Could you check a few things on this model? Use its own coordinates, in mm. Face numbers are marked on the shaded views. A direction names the side the tool comes from. Coordinates: 2 decimals unless noted, no trailing zeros. Loops run counter-clockwise (first coordinate to the right, second up) from the corner with the lowest first, then second, coordinate; pieces in that order, holes last. Notation, with made-up numbers: M 1,62 L 29,62 A38 cw 29,100 Z; hole C 54,-1.75 d7. An arc over 180 degrees is marked long. Use one line per item in the form item = value. Start each with the question number.
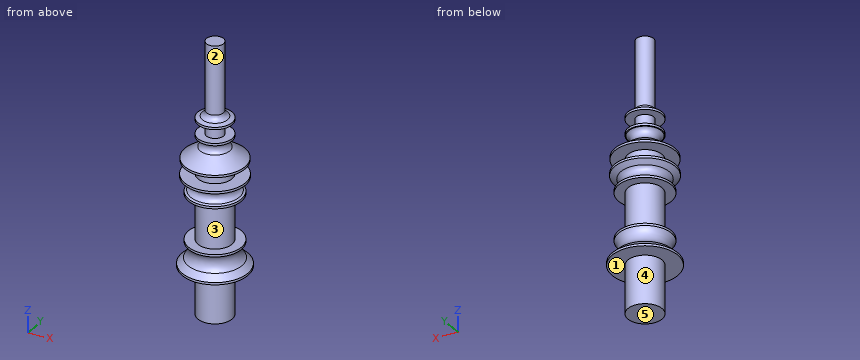
```python
from build123d import *

# Parameters (mm, degrees)
SKETCH1_R           = 14.999999999999998
BOSS_EXTRUDE1_DEPTH = 235.00000000000006
FILLET2_R           = 10
SKETCH4_W           = 104.26000000000013
SKETCH4_H           = 22.69462593232808
SKETCH10_R          = 15
BOSS_EXTRUDE2_DEPTH = 10
SCALE1_SCALE        = 1.9329
BOSS_EXTRUDE3_START = 40
SKETCH11_R          = 28.993500000000004
BOSS_EXTRUDE3_DEPTH = 40
FILLET3_R           = 10
FILLET5_R           = 10
FILLET6_R           = 10
FILLET7_R           = 10
SCALE2_SCALE        = 1.5
SKETCH12_R          = 43.49025000000001
CUT_EXTRUDE1_DEPTH  = 33.369805
SKETCH13_R          = 43.49025000000001
CUT_EXTRUDE2_DEPTH  = 20


with BuildPart() as part:
    # Sketch1 → Boss-Extrude1 (new body)
    with BuildSketch(Plane.XY):
        Circle(SKETCH1_R)
    extrude(amount=BOSS_EXTRUDE1_DEPTH)

    # Sketch2 → Revolve1 (revolve)
    with BuildSketch(Plane(origin=(0, 0, 0), x_dir=(1, 0, 0), z_dir=(0, 1, 0))):
        Polygon((0, -112.54820823836592), (0, -13.4987966999347), (11.119928350948882, -13.4987966999347), (11.119928350948882, -39.9), (15.000000000000005, -39.9), (28.84535837615048, -39.89999999999999), (28.845358376150482, -41.9), (16.269055666837332, -53.905209320131334), (23.203846346706012, -60.84), (23.203846346706015, -62.84), (7.5, -62.84), (7.4999999999999964, -102.74), (23.203846346706012, -102.74), (23.203846346706012, -104.74), (7.499999999999994, -112.54820823836592), align=None)
    revolve(axis=Axis((0, 0, 112.54820823836592), (0, 0, -1)))

    # Fillet2
    # the kernel refuses this fillet: 10 mm, written as the material it adds along each edge
    with BuildSketch(Plane(origin=(0, 0, 53.905209320131334), x_dir=(1, 0, 0), z_dir=(0, 1, 0))) as fillet2_piece_1:
        with BuildLine():
            CenterArc((30.57076321680232, -0.17250291395021122), FILLET2_R, 133.66910726980632, 88.8805373351795)
            Line((23.665838203316056, 7.060892592873103), (23.527739703046333, 7.205560503009572))
            Line((23.527739703046333, 7.205560503009572), (16.130957166567608, 0.1446679101364694))
            Line((16.130957166567608, 0.1446679101364694), (16.127634310600023, -0.14142135623730923))
            ThreePointArc((16.127634310600023, -0.14142135623730923), (19.595029650534364, -3.608816696171644), (23.05650800930409, -7.070036435187042))
            Line((23.05650800930409, -7.070036435187042), (23.203846346706015, -6.934790679868669))
        make_face()
    revolve(axis=Axis((0, 0, 53.905209320131334), (0, 0, -1)))
    with BuildSketch(Plane(origin=(0, 0, 108.81908605423119), x_dir=(1, 2.8e-16, 0), z_dir=(-2.8e-16, 1, 0))) as fillet2_piece_2:
        with BuildLine():
            CenterArc((14.999999999999998 + FILLET2_R, -FILLET2_R * 0.619575560585), FILLET2_R, 116.43731334282423, 63.56268665717579)
            Line((14.999999999999998 + FILLET2_R * 0.554781591202, FILLET2_R * 0.275846445214), (14.999999999999998 + FILLET2_R * 0.545877223026, FILLET2_R * 0.293754885329))
            Line((14.999999999999998 + FILLET2_R * 0.545877223026, FILLET2_R * 0.293754885329), (14.999999999999998 - FILLET2_R * 0.02, FILLET2_R * 0.0123915112117))
            Line((14.999999999999998 - FILLET2_R * 0.02, FILLET2_R * 0.0123915112117), (14.999999999999998 - FILLET2_R * 0.02, -FILLET2_R * 0.619575560585))
            Line((14.999999999999998 - FILLET2_R * 0.02, -FILLET2_R * 0.619575560585), (15, -FILLET2_R * 0.619575560585))
        make_face()
    revolve(axis=Axis((0, 0, 108.81908605423119), (0, 0, -1)))

    # Sketch3 → Revolve2 (revolve)
    with BuildSketch(Plane(origin=(0, 0, 0), x_dir=(0, 0, -1), z_dir=(1, 0, 0)), mode=Mode.PRIVATE) as revolve2_sk:
        Polygon((-130.74, 0), (-130.73999999999998, 14), (-128.73999999999995, 14), (-119.92783449185274, 1.1e-14), align=None)
    revolve(revolve2_sk.sketch.rotate(Axis((0, 1.1e-14, 119.92783449185274), (0, -1.02e-15, 1)), 90), axis=Axis((0, 1.1e-14, 119.92783449185274), (0, -1.02e-15, 1)))

    # Sketch4 → Cut-Revolve1 (revolve, cut)
    with BuildSketch(Plane(origin=(0, 0, 0), x_dir=(0, 0, -1), z_dir=(1, 0, 0)), mode=Mode.PRIVATE) as cut_revolve1_sk:
        with Locations((-182.87, -18.84731296616404)):
            Rectangle(SKETCH4_W, SKETCH4_H)
    revolve(cut_revolve1_sk.sketch.rotate(Axis((0, 0, 235.00000000000006), (0, 0, -1)), 90), axis=Axis((0, 0, 235.00000000000006), (0, 0, -1)), mode=Mode.SUBTRACT)

    # Sketch6 → Revolve4 (revolve)
    with BuildSketch(Plane(origin=(0, 0, 0), x_dir=(1, 0, 0), z_dir=(0, 1, 0))):
        Polygon((1.514e-14, -147.73999999999998), (1.829e-14, -173.48215721635322), (-14.999999999999986, -168.74), (-14.999999999999986, -166.74), (-7.589567298836239, -166.74), (-7.589567298836239, -154.73999999999998), (-14.999999999999986, -154.73999999999998), (-14.999999999999982, -152.73999999999998), align=None)
    revolve(axis=Axis((1.514e-14, 0, 147.73999999999998), (1.2e-16, 0, 1)))

    # Sketch8 → Revolve5 (revolve)
    with BuildSketch(Plane(origin=(0, 0, 0), x_dir=(0, 0, -1), z_dir=(1, 0, 0)), mode=Mode.PRIVATE) as revolve5_sk:
        Polygon((-152.73999999999998, 0), (-103.74000000000001, 0), (-117.74, 26.59546670677199), (-119.74, 26.59546670677199), (-119.74, 7.34766847272492), (-131.74, 7.34766847272492), (-131.74, 26.32680255189654), (-133.74, 26.32680255189654), align=None)
    revolve(revolve5_sk.sketch.rotate(Axis((0, 0, 152.73999999999998), (0, 0, -1)), 90), axis=Axis((0, 0, 152.73999999999998), (0, 0, -1)))

    # Sketch10 → Boss-Extrude2 (add)
    with BuildSketch(Plane.XY.offset(130.73999999999992)):
        with Locations(Location((0, 0, 0), (0, 0, 180))):
            Circle(SKETCH10_R)
    extrude(amount=BOSS_EXTRUDE2_DEPTH)


with BuildPart() as part_1:
    # Scale1: scaled about (0, 0, 88.197821602)
    add(part.part.scale(SCALE1_SCALE).moved(Location((0, 0, -82.27974777250581))))

    # Sketch11 → Boss-Extrude3 (add)
    with BuildSketch(Plane(origin=(0, 0, -82.27974777267455), x_dir=(-1, 0, 0), z_dir=(0, 0, -1)).offset(BOSS_EXTRUDE3_START)):
        Circle(SKETCH11_R)
    extrude(amount=-BOSS_EXTRUDE3_DEPTH)

    # Fillet3
    fillet3_edges = [part_1.edges().sort_by_distance(p)[0] for p in [
        (-29.95619321315706, -5.5e-15, 134.00840315083104),
    ]]
    fillet(fillet3_edges, radius=FILLET3_R)

    # Fillet5
    fillet5_edges = [part_1.edges().sort_by_distance(p)[0] for p in [
        (14.496749999993185, 4.19492707e-09, 248.4608560692405),
    ]]
    fillet(fillet5_edges, radius=FILLET5_R)

    # Fillet6
    # the kernel refuses this fillet: 10 mm, written as the material it adds along each edge
    with BuildSketch(Plane(origin=(-2.381562e-11, -3.695293e-11, 208.1191482274964), x_dir=(-1.0, 2.5486940639204283e-12, 0), z_dir=(-2.5486940639204283e-12, -1.0, 0))) as fillet6_piece_1:
        with BuildLine():
            CenterArc((24.364379904655884, 7.2517155656861405), FILLET6_R, 189.3328180990746, 62.23223307800339)
            Line((14.496750000023814, 5.630025069564624), (14.299397401931174, 5.597591259642201))
            ThreePointArc((14.299397401931174, 5.597591259642201), (14.296750000023817, 2.815012534782312), (14.296749999976186, 0))
            Line((14.296749999976186, 0), (14.433504446772817, -0.1897366596101051))
            Line((14.433504446772817, -0.1897366596101051), (21.13885669128414, -2.4248540744291063))
            Line((21.13885669128414, -2.4248540744291063), (21.202102244487506, -2.235117414819001))
        make_face()
    revolve(axis=Axis((-2.381562e-11, -3.695293e-11, 208.1191482274964), (0, 0, -1)))

    # Fillet7
    # the kernel refuses this fillet: 10 mm, written as the material it adds along each edge
    with BuildSketch(Plane(origin=(0, 0, 202.48912315793177), x_dir=(1, 2.8e-16, 0), z_dir=(-2.8e-16, 1, 0))) as fillet7_piece_1:
        with BuildLine():
            CenterArc((30.840499091800684, -0.5370158996013572), FILLET7_R, 125.81790747161939, 125.7471437054586)
            Line((24.988387693610907, 7.571793642074738), (24.40317655379193, 8.382674596242339))
            Line((24.40317655379193, 8.382674596242339), (13.911538860181022, 0.810880954167601))
            Line((13.911538860181022, 0.810880954167601), (13.509987009536637, -0.16216904961120804))
            ThreePointArc((13.509987009536637, -0.16216904961120804), (20.885874478501762, -8.813825782452454), (27.36199366561547, -10.972532178157024))
            Line((27.36199366561547, -10.972532178157024), (27.678221431632306, -10.023848880106499))
        make_face()
    revolve(axis=Axis((0, 0, 202.48912315793177), (0, 0, -1)), revolution_arc=180)
    with BuildSketch(Plane(origin=(0, 0, 202.48912315793177), x_dir=(-1, -1.8e-16, 0), z_dir=(1.8e-16, -1, 0))) as fillet7_piece_2:
        with BuildLine():
            CenterArc((30.84049909180068, -0.5370158996013572), FILLET7_R, 125.81790747161942, 125.74714370545857)
            Line((24.988387693610896, 7.571793642074738), (24.40317655379192, 8.382674596242339))
            Line((24.40317655379192, 8.382674596242339), (13.911538860181022, 0.810880954167601))
            Line((13.911538860181022, 0.810880954167601), (13.509987009536832, -0.16216904961237333))
            ThreePointArc((13.509987009536832, -0.16216904961237333), (20.885874478435156, -8.813825782430257), (27.361993665615465, -10.972532178157024))
            Line((27.361993665615465, -10.972532178157024), (27.678221431632302, -10.023848880106499))
        make_face()
    revolve(axis=Axis((0, 0, 202.48912315793177), (0, 0, -1)), revolution_arc=180)


with BuildPart() as part_2:
    # Scale2: scaled about (1e-08, -3.6e-08, 74.121527206)
    add(part_1.part.scale(SCALE2_SCALE).moved(Location((-5e-09, 1.8e-08, -37.060763603))))

    # Sketch12 → Cut-Extrude1 (cut)
    with BuildSketch(Plane(origin=(0, 0, -220.4803849628567), x_dir=(-1, 0, 0), z_dir=(0, 0, -1))):
        Circle(SKETCH12_R)
    extrude(amount=-CUT_EXTRUDE1_DEPTH, mode=Mode.SUBTRACT)

    # Sketch13 → Cut-Extrude2 (cut)
    with BuildSketch(Plane(origin=(0, 0, -187.11057996285672), x_dir=(-1, 0, 0), z_dir=(0, 0, -1))):
        Circle(SKETCH13_R)
    extrude(amount=-CUT_EXTRUDE2_DEPTH, mode=Mode.SUBTRACT)


solid = part_2.part
```
Item 1: I want a section at B-B (y = 50). Count the separate pieces of the cut face and the enclosed holes in it, plus the area to 3 significant figures.
Item 2: I want a section at A-A (z = 405). Write out the boundary of the cut face in (x, y), plus the area to 3 significant figures.
Item 3: I want a section at C-C (z = 52). Write out the boundary of the cut face in (x, y), plus the area to 3 significant figures.
Item 4: For the marked faces 4 and 5, which set-ups out of +Z, -Z, +X, -X, +Y, -Y let a thin tool reach every point of the face, with its end or its side?
Item 5: I'm going to push flat-ended pins straight in: P1, Ø5, axis at x = 47, y = 9.5, coming from the -Z side; P2, Ø3, axis at x = -31.5, z = -79.5, coming from the -Y side; P3, Ø3, axis at x = -22, y = 57.5, coming from the +Z side. Where does each tip first touch, or does it pass through?
Item 6: Thinking about a two-plate mould opening in Z: for the marked faces 1, 2 and 3, which applies, pulls with the +Z half, pulls with the -Z half, needs draft (parallel to the pull), parting line crosses it, or undercut?
Item 7: Please list where these lines run through material, in increasing order: line 1 along Z through (x, y) = (-6, -39); line 2 along Z through (x, y) = (-39.5, -11.5); line 3 along Z through (x, y) = (-4, 28).
Worked answers:
q1.separate_pieces = 3
q1.enclosed_holes = 0
q1.area = 11,500 mm²
q2.outline = C 0,0 d43.49
q2.area = 1,490 mm²
q3.outline = C 0,0 d86.98
q3.area = 5,940 mm²
q4.face_4 = -Z
q4.face_5 = -Z, +X, -X, +Y, -Y
q5.P1 = -44.8
q5.P2 = -31.49
q5.P3 = 239.02
q6.face_1 = pulls with the -Z half
q6.face_2 = needs draft
q6.face_3 = undercut
q7.line_1 = -167.11 to 253.89, 280.85 to 288.17, 322.96 to 330.03
q7.line_2 = -167.11 to 252.68, 281.58 to 288.17, 322.96 to 329.5
q7.line_3 = -167.11 to 288.17, 322.96 to 334.23
